The listing builds one solid part. Answer for the finished solid, in the listing's coordinates (mm). A direction names the side the tool comes from. Give positions to 0.01 mm unless a question says otherwise; leave off trailing zeros. Order: outer loops, then holes, each group sorted by start corner. A loop starts at its lowest first (then second) coordinate and runs counter-clockwise, first axis right, second up. Notation, with made-up numbers: (-29.5, 57) -> (-21.5, 57) arc R37 ccw to (-21.5, 93) -> close; hole circle Ø3 at (20, 25.25). An arc over 180 degrees is marked (long way). One line per question, with ' | ' between items. Start each with the question number.
```python
from build123d import *

# Parameters (mm, degrees)
F1_DEPTH = 5
F2_R     = 5
F3_DEPTH = 7
F5_R     = 2.5
F6_DEPTH = 12.001
F7_W     = 15.130732
F7_H     = 3
F8_DEPTH = 3


with BuildPart() as f1:
    # F0 (on Top) → F1 (new body)
    with BuildSketch(Plane.XY):
        with BuildLine():
            ThreePointArc((7.75, 13.423394), (5.931593, 14.320133), (4.011695, 14.97185))
            ThreePointArc((4.011695, 14.97185), (0, 15.5), (-4.011695, 14.97185))
            ThreePointArc((-4.011695, 14.97185), (-5.931593, 14.320133), (-7.75, 13.423394))
            ThreePointArc((-7.75, 13.423394), (-10.960155, 10.960155), (-13.423394, 7.75))
            ThreePointArc((-13.423394, 7.75), (-14.320133, 5.931593), (-14.97185, 4.011695))
            ThreePointArc((-14.97185, 4.011695), (-15.5, 0), (-14.97185, -4.011695))
            ThreePointArc((-14.97185, -4.011695), (-14.320133, -5.931593), (-13.423394, -7.75))
            ThreePointArc((-13.423394, -7.75), (-10.960155, -10.960155), (-7.75, -13.423394))
            ThreePointArc((-7.75, -13.423394), (-5.931593, -14.320133), (-4.011695, -14.97185))
            ThreePointArc((-4.011695, -14.97185), (0, -15.5), (4.011695, -14.97185))
            ThreePointArc((4.011695, -14.97185), (5.931593, -14.320133), (7.75, -13.423394))
            ThreePointArc((7.75, -13.423394), (10.960155, -10.960155), (13.423394, -7.75))
            ThreePointArc((13.423394, -7.75), (14.320133, -5.931593), (14.97185, -4.011695))
            ThreePointArc((14.97185, -4.011695), (15.367395, -2.023156), (15.5, 0))
            ThreePointArc((15.5, 0), (15.367395, 2.023156), (14.97185, 4.011695))
            ThreePointArc((14.97185, 4.011695), (14.320133, 5.931593), (13.423394, 7.75))
            ThreePointArc((13.423394, 7.75), (10.960155, 10.960155), (7.75, 13.423394))
        make_face()
        with BuildLine():
            ThreePointArc((-4.011695, 14.97185), (0, 15.5), (4.011695, 14.97185))
            Line((4.011695, 14.97185), (0.499976, 25.495098))
            ThreePointArc((0.499976, 25.495098), (0, 25.5), (-0.499976, 25.495098))
            Line((-0.499976, 25.495098), (-4.011695, 14.97185))
        make_face()
        with BuildLine():
            Line((17.67422, 18.381293), (7.75, 13.423394))
            ThreePointArc((7.75, 13.423394), (10.960155, 10.960155), (13.423394, 7.75))
            Line((13.423394, 7.75), (18.381293, 17.67422))
            ThreePointArc((18.381293, 17.67422), (18.031223, 18.031223), (17.67422, 18.381293))
        make_face()
        with BuildLine():
            ThreePointArc((-13.423394, 7.75), (-10.960155, 10.960155), (-7.75, 13.423394))
            Line((-7.75, 13.423394), (-17.67422, 18.381293))
            ThreePointArc((-17.67422, 18.381293), (-18.031223, 18.031223), (-18.381293, 17.67422))
            Line((-18.381293, 17.67422), (-13.423394, 7.75))
        make_face()
        with BuildLine():
            Line((25.495098, 0.499976), (14.97185, 4.011695))
            ThreePointArc((14.97185, 4.011695), (15.367395, 2.023156), (15.5, 0))
            ThreePointArc((15.5, 0), (15.367395, -2.023156), (14.97185, -4.011695))
            Line((14.97185, -4.011695), (25.495098, -0.499976))
            ThreePointArc((25.495098, -0.499976), (25.5, 0), (25.495098, 0.499976))
        make_face()
        with BuildLine():
            ThreePointArc((-14.97185, -4.011695), (-15.5, 0), (-14.97185, 4.011695))
            Line((-14.97185, 4.011695), (-25.495098, 0.499976))
            ThreePointArc((-25.495098, 0.499976), (-25.5, 0), (-25.495098, -0.499976))
            Line((-25.495098, -0.499976), (-14.97185, -4.011695))
        make_face()
        with BuildLine():
            ThreePointArc((-7.75, -13.423394), (-10.960155, -10.960155), (-13.423394, -7.75))
            Line((-13.423394, -7.75), (-18.381293, -17.67422))
            ThreePointArc((-18.381293, -17.67422), (-18.031223, -18.031223), (-17.67422, -18.381293))
            Line((-17.67422, -18.381293), (-7.75, -13.423394))
        make_face()
        with BuildLine():
            Line((18.381293, -17.67422), (13.423394, -7.75))
            ThreePointArc((13.423394, -7.75), (10.960155, -10.960155), (7.75, -13.423394))
            Line((7.75, -13.423394), (17.67422, -18.381293))
            ThreePointArc((17.67422, -18.381293), (18.031223, -18.031223), (18.381293, -17.67422))
        make_face()
        with BuildLine():
            ThreePointArc((4.011695, -14.97185), (0, -15.5), (-4.011695, -14.97185))
            Line((-4.011695, -14.97185), (-0.499976, -25.495098))
            ThreePointArc((-0.499976, -25.495098), (0, -25.5), (0.499976, -25.495098))
            Line((0.499976, -25.495098), (4.011695, -14.97185))
        make_face()
    extrude(amount=F1_DEPTH)

    # F2 (on face) → F3 (join)
    with BuildSketch(Plane.XY.offset(5)):
        Circle(F2_R)
    extrude(amount=F3_DEPTH)

    # F5 (on face) → F6 (cut, through all)
    with BuildSketch(Plane.XY.offset(12)):
        Circle(F5_R)
    extrude(amount=-F6_DEPTH, mode=Mode.SUBTRACT)

    # F7 (on face) → F8 (cut)
    with BuildSketch(Plane.XY.offset(12)):
        with Locations((0.217972, 0)):
            Rectangle(F7_W, F7_H)
    extrude(amount=-F8_DEPTH, mode=Mode.SUBTRACT)


solid = f1.part
```
(1) The part is cut by section D-D on z = 7.25. Determine the outline of the cut face in (x, y), plus the area to 3 significant figures.
(2) Given P1, Ø0.8, axis at x = -4, z = 10, coming from the -Y side; P2, Ø3, axis at x = 3.5, z = 11, coming from the -Y side; P3, Ø2, axis at x = -3.5, z = 11, coming from the +Y side, each flat-ended and moving along its own axis, determine where each tip first touches the part or whether it passes through.
(3) The part is cut by section B-B on y = -10. Determine the outline of the cut face in (x, z), plus the area to 3 significant figures.
(4) The part is cut by section C-C on x = 22. Determine the outline of the cut face in (y, z), plus the area to 3 significant figures.
(5) For faces 4 (the face through (12.782, 15.937, 2.465)), 5 (the face through (12.643, -15.868, 2.465)), 6 (the face through (3, 1.5, 11)), 7 (the face through (-15.937, 12.782, 2.465)), 8 (the face through (4.77, 1.5, 8.45)), determine the directions among +Z, -Z, +X, -X, +Y, -Y from which every point of the face is accessible in a straight line to the end or side of a thin tool.
(6) Determine the mould class of faces 1 (the face through (2.28, 20.16, 2.46)), 2 (the face through (3, 0, 9)), 3 (the face through (14.31, -5.96, 2.46)) for opening direction X: pulls with the +X half, pulls with the -X half, needs draft (parallel to the pull), parting line crosses it, or undercut.
(7) Consider line 1 (Y direction, x = 0, z = 5.5); line 2 (X direction, y = 0, z = 2.75). Determine where each line is inside the solid, lowest interval first.
Result sheet:
1) outline: circle Ø10 at (0, 0); hole circle Ø5 at (0, 0) | area: 58.9 mm^2
2) P1: stops at y = -3.47 | P2: stops at y = -4.58 | P3: stops at y = 4.33
3) outline: (-14.55, 0) -> (14.55, 0) -> (14.55, 5) -> (-14.55, 5) -> close | area: 145 mm^2
4) outline: (-1.67, 0) -> (1.67, 0) -> (1.67, 5) -> (-1.67, 5) -> close | area: 16.7 mm^2
5) face 4: +Z, -Z, +Y | face 5: +Z, -Z, -Y | face 6: +Z, +X, -X | face 7: +Z, -Z, -X | face 8: +Z
6) face 1: undercut | face 2: needs draft | face 3: pulls with the +X half
7) line 1: y = -5 to -2.5, 2.5 to 5 | line 2: x = -25.5 to -2.5, 2.5 to 25.5
